Input: part model. Units: mm. Frame: model coordinates. Give positions to 0.01 mm unless a question says otherwise; leave off trailing zeros. Loops run counter-clockwise (first coordinate to the right, second up) from the corner with the lowest first, then second, coordinate; pieces in that order, holes last. Notation, with made-up numbers: M -0.75,-18 L 41.25,-18 A16 ccw 41.25,6 Z; hole C 72,-26.5 d5. An arc over 180 degrees is marked long. Use CSV: the item, a comma, the result in double quotes. Start each with the question number.
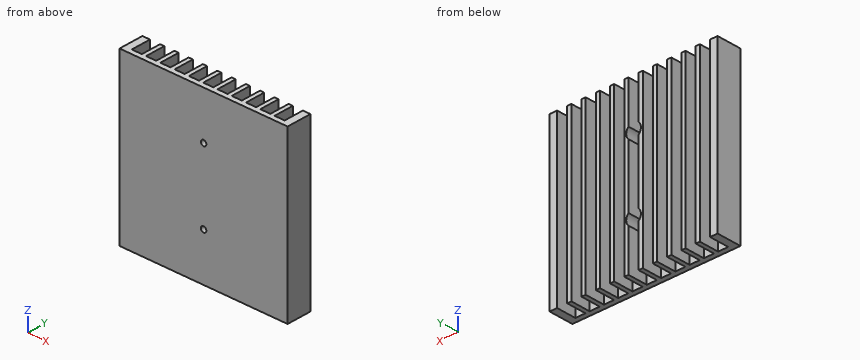
from build123d import *

# Parameters (mm, degrees)
SKETCH1_W           = 101.6
SKETCH1_H           = 101.6
BOSS_EXTRUDE1_DEPTH = 14.986
SKETCH2_W           = 6.096
SKETCH2_H           = 11.938
CUT_EXTRUDE1_DEPTH  = 115.576525502
SKETCH3_R           = 1.651
CUT_EXTRUDE2_DEPTH  = 74.38842004
CUT_EXTRUDE3_START  = -3.048
SKETCH3_3_R         = 4.445
SKETCH3_3_R_2       = 1.651
CUT_EXTRUDE3_DEPTH  = 71.34042004


with BuildPart() as part:
    # Sketch1 → Boss-Extrude1 (new body)
    with BuildSketch(Plane(origin=(0, 0, 0), x_dir=(1, 0, 0), z_dir=(0, 1, 0))):
        Rectangle(SKETCH1_W, SKETCH1_H)
    extrude(amount=BOSS_EXTRUDE1_DEPTH)

    # Sketch2 → Cut-Extrude1 (cut, through all)
    with BuildSketch(Plane.XY.offset(50.8)):
        with Locations((43.18, 9.017)):
            Rectangle(SKETCH2_W, SKETCH2_H)
        with Locations((34.544, 9.017)):
            Rectangle(SKETCH2_W, SKETCH2_H)
        with Locations((25.908, 9.017)):
            Rectangle(SKETCH2_W, SKETCH2_H)
        with Locations((17.272, 9.017)):
            Rectangle(SKETCH2_W, SKETCH2_H)
        with Locations((8.636, 9.017)):
            Rectangle(SKETCH2_W, SKETCH2_H)
        with Locations((0, 9.017)):
            Rectangle(SKETCH2_W, SKETCH2_H)
        with Locations((-8.636, 9.017)):
            Rectangle(SKETCH2_W, SKETCH2_H)
        with Locations((-17.272, 9.017)):
            Rectangle(SKETCH2_W, SKETCH2_H)
        with Locations((-25.908, 9.017)):
            Rectangle(SKETCH2_W, SKETCH2_H)
        with Locations((-34.544, 9.017)):
            Rectangle(SKETCH2_W, SKETCH2_H)
        with Locations((-43.18, 9.017)):
            Rectangle(SKETCH2_W, SKETCH2_H)
    extrude(amount=-CUT_EXTRUDE1_DEPTH, mode=Mode.SUBTRACT)

    # Sketch3 → Cut-Extrude2 (cut, through all)
    with BuildSketch(Plane.XZ):
        with Locations(Location((0, 22.225, 0), (0, 0, 270))):
            Circle(SKETCH3_R)
        with Locations(Location((0, -22.225, 0), (0, 0, 270))):
            Circle(SKETCH3_R)
    extrude(amount=-CUT_EXTRUDE2_DEPTH, mode=Mode.SUBTRACT)

    # Sketch3<3> → Cut-Extrude3 (cut, through all)
    # profile 1 of 2: a face of its own
    with BuildSketch(Plane.XZ.offset(CUT_EXTRUDE3_START)):
        with Locations((0, 22.225)):
            Circle(SKETCH3_3_R)
        with Locations(Location((0, 22.225, 0), (0, 0, 270))):
            Circle(SKETCH3_3_R_2, mode=Mode.SUBTRACT)
    # profile 2 of 2: a face of its own
    with BuildSketch(Plane.XZ.offset(CUT_EXTRUDE3_START)):
        with Locations((0, -22.225)):
            Circle(SKETCH3_3_R)
        with Locations(Location((0, -22.225, 0), (0, 0, 270))):
            Circle(SKETCH3_3_R_2, mode=Mode.SUBTRACT)
    extrude(amount=-CUT_EXTRUDE3_DEPTH, mode=Mode.SUBTRACT)


solid = part.part
Item 1: Section A-A (x = 0). Output: boundary loops of the cut face in (y, z), then the cut area to 3 significant figures.
Item 2: First-contact query: pin 1 Ø5 at (x, z) = (-9, 17.5) entering from +Y; pin 2 Ø1 at (x, y) = (36.5, 5.5) entering from +Z. Flat tips, straight axial feed; report the tip coordinate or a pass-through.
Item 3: Section B-B (y = 12.5). State how many separate pieces and enclosed holes the cut face has, then the cut area to 3 significant figures.
Item 4: Section C-C (x = -34). Output: boundary loops of the cut face in (y, z).
Item 5: Material intervals for line 1 (Y direction, x = 17, z = -44.5), sorted ascending.
Recorded:
1,outline,"M 0,-50.8 L 3.05,-50.8 L 3.05,-23.88 L 0,-23.88 Z; M 0,-20.57 L 3.05,-20.57 L 3.05,20.57 L 0,20.57 Z; M 0,23.88 L 3.05,23.88 L 3.05,50.8 L 0,50.8 Z"
1,area,"290 mm²"
2,pin 1,"y = 3.05"
2,pin 2,"through"
3,separate pieces,"12"
3,enclosed holes,"0"
3,area,"3,480 mm²"
4,outline,"M 0,-50.8 L 3.05,-50.8 L 3.05,50.8 L 0,50.8 Z"
5,line 1,"0 to 3.05"
